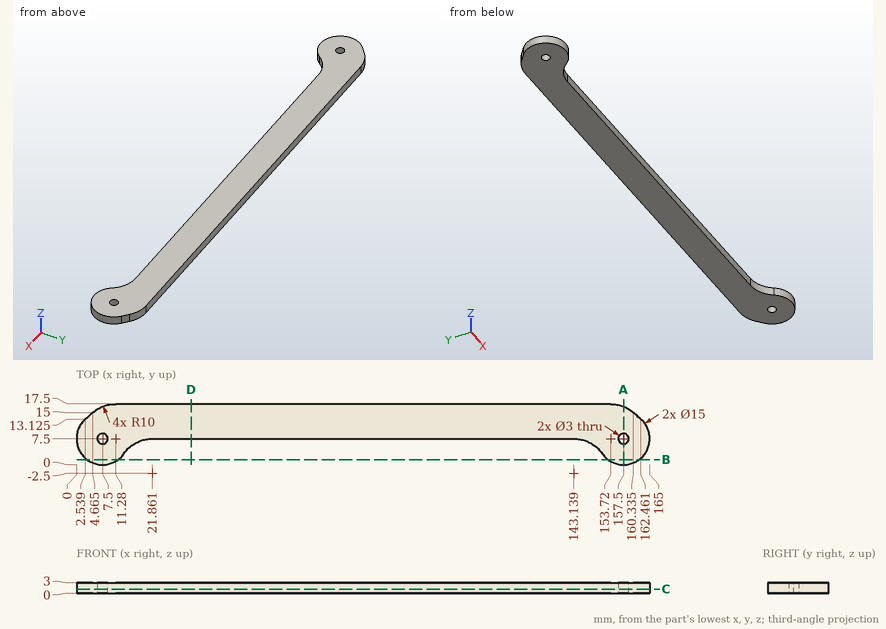
Design review of the part shown in the three views and the two pictorial views. Dimensions are in mm from the part's minimum x, y and z. Round coordinates to 2 decimals unless told otherwise and drop trailing zeros. Loops run counter-clockwise (first coordinate to the right, second up) from the corner with the lowest first, then second, coordinate; pieces in that order, holes last. Notation, with made-up numbers: (66.5, -25.75) - (116.5, -25.75) arc R6 cw to (116.5, -19.75) - close; hole circle Ø3 at (84, -27.75). An arc over 180 degrees is marked (long way). Write each question's results on one line, items separated by ' | '. Start each with the question number.
Q1. Take a section at A-A on x = 157.5. Give the boundary of the cut face in (y, z).
Q2. Take a section at C-C on z = 1.2. Give the boundary of the cut face in (x, y) (1 decimal).
Q3. Insertion check: P1, Ø3, axis at x = 43, y = 7.5, coming from the -Z side; P2, Ø1.5, axis at x = 18, z = 2.5, coming from the -Y side; P3, Ø1.5, axis at x = 74.5, z = 1.5, coming from the -Y side. Each pin has a flat end and moves straight along its axis. Give the tip position at first contact, or say it passes through.
Q4. Take a section at D-D on x = 33. Give the boundary of the cut face in (y, z), plus the area to 3 significant figures.
Q5. Take a section at B-B on y = 1.5. Give the boundary of the cut face in (x, z).
Q6. Wall thickness on line 1 along X through (y, z) = (7.75, 0.8) (1 decimal); line 2 along Y through (x, z) = (134, 2.3); line 3 along X through (y, z) = (2.5, 0.6): over which ranges is each line inside the solid? List them lowest first. Write a range as [from, to].
Data:
1) outline: (0, 0) - (6, 0) - (6, 3) - (0, 3) - close; (9, 0) - (16.76, 0) - (16.76, 3) - (9, 3) - close
2) outline: (2.5, 13.1) arc R7.5 ccw (long way) to (13.7, 3.2) arc R10 cw to (21.9, 7.5) - (143.1, 7.5) arc R10 cw to (151.3, 3.2) arc R7.5 ccw (long way) to (162.5, 13.1) - (160.3, 15) arc R10 ccw to (153.7, 17.5) - (11.3, 17.5) arc R10 ccw to (4.7, 15) - close; hole circle Ø3 at (7.5, 7.5); hole circle Ø3 at (157.5, 7.5)
3) P1: stops at z = 0 | P2: stops at y = 6.37 | P3: stops at y = 7.5
4) outline: (7.5, 0) - (17.5, 0) - (17.5, 3) - (7.5, 3) - close | area: 30.0 mm²
5) outline: (3, 0) - (12, 0) - (12, 3) - (3, 3) - close; (153, 0) - (162, 0) - (162, 3) - (153, 3) - close
6) line 1: x = [0, 6], [9, 156], [159, 165] | line 2: y = [7.5, 17.5] | line 3: x = [1.91, 13.09], [151.91, 163.09]
